Can you work these out from the drawing? Everything is in mm from the part's minimum corner. Coordinates: 2 decimals unless noted, no trailing zeros. Write each loop counter-clockwise with the first axis right and the second up, starting at its lowest first coordinate (ties: lowest second). Pieces come first, ordered by that corner, then holes. Notation, with made-up numbers: M 23,-8.75 L 55,-8.75 A18 cw 55,4.25 Z; hole C 87.5,5.5 d7. An arc over 180 degrees is marked long. Answer as a JSON object with one key per item and string values. Group by question number.
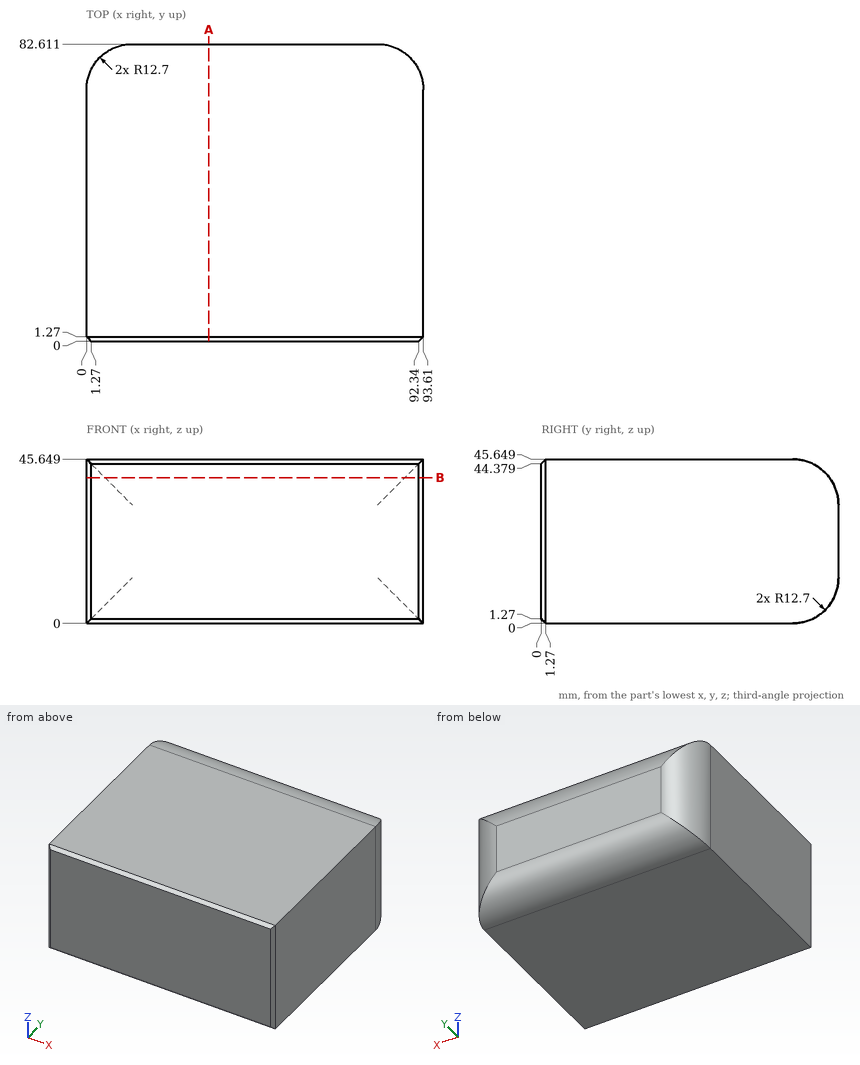
Q1. If we section it at A-A on x = 34: List the corners of the cut face in (y, z) for me.
Q2. Please list where these lines run through material, in increasing order: L1, parallel to Y at x = 38, z = 12; L2, parallel to Z at x = 70, y = 72.5; L3, parallel to Y at x = 34, z = 36.
Q3. If we section it at B-B on z = 40.5: List the corners of the cut face in (x, y) for me, and give its area (3 significant figures).
Q4. Will these pins go through, and if not, where does the flat tip stop? pin 1 (8 mm diameter, centred on x = 15.5, z = 5.5, fed in from +Y); pin 2 (1.5 mm diameter, centred on x = 19.5, z = 39.5, fed in from +Y).
Reply:
{
 "1": {"outline": "M 0,1.27 L 1.27,0 L 69.91,0 A12.7 ccw 82.61,12.7 L 82.61,32.95 A12.7 ccw 69.91,45.65 L 1.27,45.65 L 0,44.38 Z"},
 "2": {"L1": "0 to 82.59", "L2": "0.27 to 45.38", "L3": "0 to 82.24"},
 "3": {"outline": "M 0,1.27 L 1.27,0 L 92.34,0 L 93.61,1.27 L 93.61,69.91 A12.7 ccw 88.46,80.12 L 5.15,80.12 A12.7 ccw 0,69.91 Z", "area": "7,470 mm^2"},
 "4": {"pin 1": "y = 82.2", "pin 2": "y = 81.21"}
}
